Design review of the part built by this model. Coordinates are the model's own, in mm. Round coordinates to 2 decimals unless told otherwise and drop trailing zeros. Loops run counter-clockwise (first coordinate to the right, second up) from the corner with the lowest first, then second, coordinate; pieces in that order, holes last. Notation, with made-up numbers: M -23,-21 L 20,-21 A30 ccw 20,11 Z; hole C 3.5,13 d1. An arc over 180 degrees is marked long. One line per item, written item: value. Start each with the question number.
Item 1: We need section A-A (x = 225). Write out the cut boundary in (y, z).
Item 2: We need section C-C (y = 43). Write out the cut boundary in (x, z).
Item 3: Clearance check with flat-ended pins moving along their axes: pin 1 (3.5 mm diameter, centred on x = -140, z = 3.5, fed in from +Y); pin 2 (12 mm diameter, centred on x = -79, z = 6, fed in from +Y); pin 3 (1 mm diameter, centred on x = -250, z = 10.5, fed in from +Y). State where each tip first meets the part, or that it passes through.
Item 4: We need section B-B (y = -14). Write out the cut boundary in (x, z), then the cut area to 3 significant figures.
Item 5: For line 1 along Y through (x, z) = (-293, 20.5); line 2 along Z through (x, y) = (-328.5, -13.5); line 3 along Y through (x, z) = (175.5, 13), list the stretches that pass through material, from the lowest coordinate up.
from build123d import *

# Parameters (mm, degrees)
F1_DEPTH = 400


with BuildPart() as f1:
    # F0 (on Right) → F1 (new body, symmetric)
    with BuildSketch(Plane.YZ):
        with BuildLine():
            ThreePointArc((36, 11.393311), (45.989188, 11.411984), (50.9784, 20.066))
            ThreePointArc((50.9784, 20.066), (41.121, 30.064983), (30.982467, 20.35117))
            ThreePointArc((30.982467, 20.35117), (32.25381, 15.179127), (36, 11.393311))
        make_face()
        with BuildLine():
            ThreePointArc((36, 11.393311), (32.25381, 15.179127), (30.982467, 20.35117))
            ThreePointArc((30.982467, 20.35117), (27.450179, 15.715402), (26.983, 9.906))
            Line((26.983, 9.906), (0, 9.906))
            Line((0, 9.906), (0, 0))
            Line((0, 0), (36, 0))
            Line((36, 0), (36, 11.393311))
        make_face()
        with BuildLine():
            Line((0, 0), (0, 9.906))
            Line((0, 9.906), (-26.983, 9.906))
            ThreePointArc((-26.983, 9.906), (-27.450179, 15.715402), (-30.982467, 20.35117))
            ThreePointArc((-30.982467, 20.35117), (-30.979417, 20.2086), (-30.9784, 20.066))
            ThreePointArc((-30.9784, 20.066), (-32.324384, 15.055212), (-36, 11.393311))
            Line((-36, 11.393311), (-36, 0))
            Line((-36, 0), (0, 0))
        make_face()
        with BuildLine():
            ThreePointArc((-30.9784, 20.066), (-30.979417, 20.2086), (-30.982467, 20.35117))
            ThreePointArc((-30.982467, 20.35117), (-49.70299, 24.952873), (-36, 11.393311))
            ThreePointArc((-36, 11.393311), (-32.324384, 15.055212), (-30.9784, 20.066))
        make_face()
    extrude(amount=F1_DEPTH, both=True)


solid = f1.part
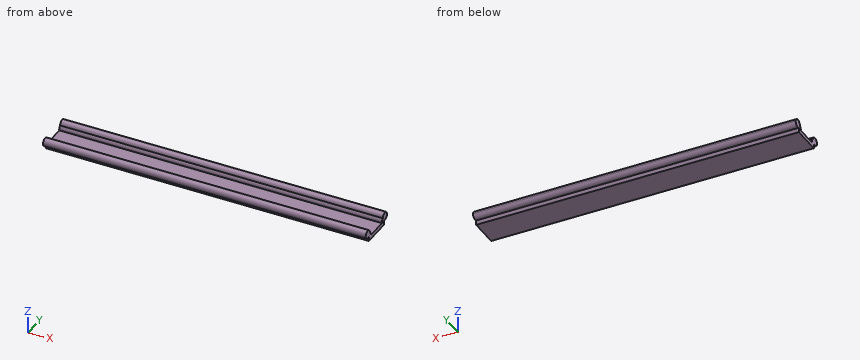
A:
1. outline: M -36,0 L 36,0 L 36,11.39 A10 ccw 50.98,20.07 A10 ccw 30.98,20.35 A10.35 ccw 26.98,9.91 L -26.98,9.91 A10.35 ccw -30.98,20.35 A10 ccw long -36,11.39 Z
2. outline: M -400,10.27 L 400,10.27 L 400,29.86 L -400,29.86 Z
3. pin 1: y = 36
3. pin 2: y = 46.89
3. pin 3: y = 45.2
4. outline: M -400,0 L 400,0 L 400,9.91 L -400,9.91 Z
4. area: 7,920 mm2
5. line 1: -50.97 to -30.99, 30.99 to 50.97
5. line 2: 0 to 9.91
5. line 3: -48.05 to -26.81, 26.81 to 48.05
